Source: CAD feature listing. Evaluate the final solid. Frame: model axes, mm. Coordinates: 2 decimals unless noted, no trailing zeros. Loops run counter-clockwise (first coordinate to the right, second up) from the corner with the lowest first, then second, coordinate; pieces in that order, holes last.
Item 1: Section query D-D, the plane y = -161. Return the cut outline in (x, z), then the cut area to 3 significant figures.
Item 2: Line query: probe 1 along Y at (x, z) = (68, 2.3); probe 2 along X at (y, z) = (-168, 2.7); probe 3 along X at (y, z) = (-120.5, 0.2). Output: solid intervals per line, ascending.
Item 3: Section query C-C, the plane y = -30.5. Return the cut outline in (x, z).
Item 4: Section query B-B, the plane y = -77. Return the cut outline in (x, z), then the cut area to 3 significant figures.
Item 5: Section query A-A, the plane x = 67.5. Return the cut outline in (y, z).
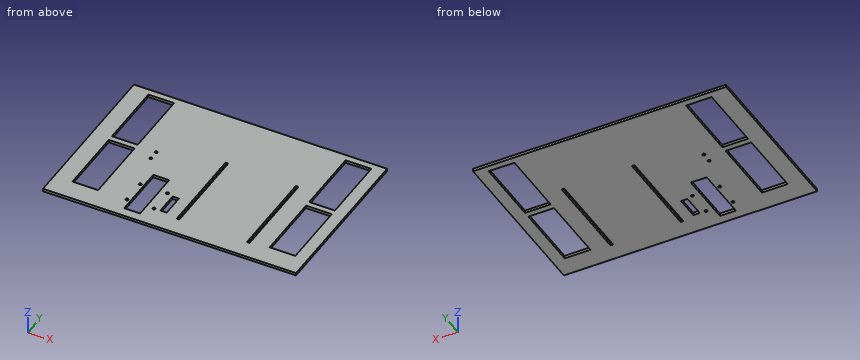
```python
from build123d import *

# Parameters (mm, degrees)
F1_W     = 285.75
F1_H     = 190.5
F1_R     = 1.5494
F1_W_2   = 18.034
F1_H_2   = 60.96
F1_W_3   = 7.226892
F1_H_3   = 25.737308
F1_W_4   = 29.083
F1_H_4   = 76.2
F1_W_5   = 3.0988
F1_H_5   = 102.414822
F2_DEPTH = 3.0988


with BuildPart() as f2:
    # F1 (on face) → F2 (new body)
    with BuildSketch(Plane.XY):
        with Locations((-38.680092, -95.25)):
            Rectangle(F1_W, F1_H)
        with Locations((-99.931192, -166.0906)):
            Circle(F1_R, mode=Mode.SUBTRACT)
        with Locations((-86.723192, -149.2377)):
            Rectangle(F1_W_2, F1_H_2, mode=Mode.SUBTRACT)
        with Locations((-69.146392, -166.0906)):
            Circle(F1_R, mode=Mode.SUBTRACT)
        with Locations((-58.674946, -153.221946)):
            Rectangle(F1_W_3, F1_H_3, mode=Mode.SUBTRACT)
        with Locations((-146.794192, -128.380313)):
            Rectangle(F1_W_4, F1_H_4, mode=Mode.SUBTRACT)
        with Locations((-110.472192, -96.5073)):
            Circle(F1_R, mode=Mode.SUBTRACT)
        with Locations((-99.931192, -138.1506)):
            Circle(F1_R, mode=Mode.SUBTRACT)
        with Locations((-69.146392, -138.1506)):
            Circle(F1_R, mode=Mode.SUBTRACT)
        with Locations((-40.252562, -118.60587)):
            Rectangle(F1_W_5, F1_H_5, mode=Mode.SUBTRACT)
        with Locations((75.973835, -128.380313)):
            Rectangle(F1_W_4, F1_H_4, mode=Mode.SUBTRACT)
        with Locations((39.046238, -118.60587)):
            Rectangle(F1_W_5, F1_H_5, mode=Mode.SUBTRACT)
        with Locations((-110.472192, -85.2932)):
            Circle(F1_R, mode=Mode.SUBTRACT)
        with Locations((-146.794192, -45.493023)):
            Rectangle(F1_W_4, F1_H_4, mode=Mode.SUBTRACT)
        with Locations((75.973835, -45.493023)):
            Rectangle(F1_W_4, F1_H_4, mode=Mode.SUBTRACT)
    extrude(amount=F2_DEPTH)


solid = f2.part
```
Verdict:
1. outline: (-181.56, 0) - (-161.34, 0) - (-161.34, 3.1) - (-181.56, 3.1) - close; (-132.25, 0) - (-95.74, 0) - (-95.74, 3.1) - (-132.25, 3.1) - close; (-77.71, 0) - (-62.29, 0) - (-62.29, 3.1) - (-77.71, 3.1) - close; (-55.06, 0) - (-41.8, 0) - (-41.8, 3.1) - (-55.06, 3.1) - close; (-38.7, 0) - (37.5, 0) - (37.5, 3.1) - (-38.7, 3.1) - close; (40.6, 0) - (61.43, 0) - (61.43, 3.1) - (40.6, 3.1) - close; (90.52, 0) - (104.19, 0) - (104.19, 3.1) - (90.52, 3.1) - close
1. area: 608 mm2
2. probe 1: y = -190.5 to -166.48, -90.28 to -83.59, -7.39 to 0
2. probe 2: x = -181.56 to -95.74, -77.71 to -41.8, -38.7 to 37.5, 40.6 to 104.19
2. probe 3: x = -181.56 to -161.34, -132.25 to -95.74, -77.71 to -41.8, -38.7 to 37.5, 40.6 to 61.43, 90.52 to 104.19
3. outline: (-181.56, 0) - (-161.34, 0) - (-161.34, 3.1) - (-181.56, 3.1) - close; (-132.25, 0) - (61.43, 0) - (61.43, 3.1) - (-132.25, 3.1) - close; (90.52, 0) - (104.19, 0) - (104.19, 3.1) - (90.52, 3.1) - close
4. outline: (-181.56, 0) - (-161.34, 0) - (-161.34, 3.1) - (-181.56, 3.1) - close; (-132.25, 0) - (-41.8, 0) - (-41.8, 3.1) - (-132.25, 3.1) - close; (-38.7, 0) - (37.5, 0) - (37.5, 3.1) - (-38.7, 3.1) - close; (40.6, 0) - (61.43, 0) - (61.43, 3.1) - (40.6, 3.1) - close; (90.52, 0) - (104.19, 0) - (104.19, 3.1) - (90.52, 3.1) - close
4. area: 686 mm2
5. outline: (-190.5, 0) - (-166.48, 0) - (-166.48, 3.1) - (-190.5, 3.1) - close; (-90.28, 0) - (-83.59, 0) - (-83.59, 3.1) - (-90.28, 3.1) - close; (-7.39, 0) - (0, 0) - (0, 3.1) - (-7.39, 3.1) - close
